Read the model definition and answer for the solid it produces. Units are mm, in the model's axes. A direction names the side the tool comes from. Give positions to 0.01 mm unless a question says otherwise; leave off trailing zeros. Order: outer loops, then holes, each group sorted by start corner. A loop starts at its lowest first (then second) coordinate and runs counter-clockwise, first axis right, second up. Notation, with made-up numbers: (-26.5, 0) - (19.5, 0) arc R20 cw to (19.5, 37) - close; hole circle Ø6 at (5.5, 38). An arc over 180 degrees is marked (long way). Use a Markdown table: item, result. Add a question column.
1. A cutting plane is placed at C-C on x = 1.25. Determine the outline of the cut face in (y, z), and give its area (3 significant figures).
2. A cutting plane is placed at A-A on y = -1.65. Determine the outline of the cut face in (x, z), and give its area (3 significant figures).
3. A cutting plane is placed at D-D on z = 6.75. Determine the outline of the cut face in (x, y).
4. For a pull along X with two mould halves and no side action, classify faces 4 (the flat face through (0, 0, 6)), 5 (the flat face through (19, 2, 3)), 6 (the flat face through (9, 0, 9.7)) as released by +X, released by -X, zero draft, split by the parting line, or undercut.
5. A cutting plane is placed at B-B on z = 4. Determine the outline of the cut face in (x, y), and give its area (3 significant figures).
6. Flat-ended cylindrical pins translate along their axes: P1, Ø1, axis at x = 19, y = 1, coming from the +Z side; P2, Ø1.5, axis at x = 7.5, y = -0.5, coming from the +Z side; P3, Ø2, axis at x = 18.5, z = 4.5, coming from the +Y side. Find the tip coordinate at first contact, or state that the pin passes through.
7. Which of the six approach directions +Z, -Z, +X, -X, +Y, -Y give full straight-line access (tool end or side, diameter ignored) to faces 1 (the flat face through (19, 0, 9)), 2 (the flat face through (19, -2.5, 6)), 3 (the flat face through (19, -2, 3))?
8. Consider L1, parallel to Z at x = 19.25, y = 1.3; L2, parallel to Y at x = 1.5, z = 5.5; L3, parallel to Z at x = 12.75, y = -2.5. Determine where each line is inside the solid, lowest interval first.
```python
from build123d import *

# Parameters (mm, degrees)
PAD_DEPTH         = 20
POCKET_DEPTH      = 2.951
POCKET_DEPTH_BACK = -2.951
PAD001_DEPTH      = 2
PAD002_DEPTH      = 0.7


with BuildPart() as part:
    # Sketch → Pad (new body)
    with BuildSketch(Plane.YZ):
        Polygon((-2.95, 0), (-2.95, 1.4), (-0.7, 1.4), (-0.7, 14.4), (0.7, 14.4), (0.7, 1.4), (2.95, 1.4), (2.95, 0), align=None)
    extrude(amount=PAD_DEPTH)

    # Sketch002 → Pocket (cut, two sides)
    with BuildSketch(Plane.XZ) as pocket_sk:
        Polygon((20, 14.4), (2.290965, 14.4), (20, 2), align=None)
    extrude(amount=-POCKET_DEPTH, mode=Mode.SUBTRACT)
    extrude(pocket_sk.sketch, amount=-POCKET_DEPTH_BACK, mode=Mode.SUBTRACT)

    # Sketch001 (on DatumPlane) → Pad001 (join)
    with BuildSketch(Plane.YZ.offset(20)):
        Polygon((-2.5, 9), (2.5, 9), (2.5, 3), (0.7, 3), (0.7, 1.4), (-0.7, 1.4), (-0.7, 3), (-2.5, 3), align=None)
    extrude(amount=-PAD001_DEPTH)

    # Sketch003 → Pad002 (join, symmetric)
    with BuildSketch(Plane.XZ):
        Polygon((20, 3), (14, 3), (20, 9), align=None)
    extrude(amount=PAD002_DEPTH, both=True)


solid = part.part
```
Output values:
| question | item | result |
|---|---|---|
| 1 | outline | (-2.95, 0) - (2.95, 0) - (2.95, 1.4) - (0.7, 1.4) - (0.7, 14.4) - (-0.7, 14.4) - (-0.7, 1.4) - (-2.95, 1.4) - close |
| 1 | area | 26.5 mm² |
| 2 | outline | (0, 0) - (20, 0) - (20, 1.4) - (0, 1.4) - close; (18, 3) - (20, 3) - (20, 9) - (18, 9) - close |
| 2 | area | 40.0 mm² |
| 3 | outline | (0, -0.7) - (13.22, -0.7) - (13.22, 0.7) - (0, 0.7) - close; (17.75, -0.7) - (18, -0.7) - (18, -2.5) - (20, -2.5) - (20, 2.5) - (18, 2.5) - (18, 0.7) - (17.75, 0.7) - close |
| 4 | face 4 | released by -X |
| 4 | face 5 | zero draft |
| 4 | face 6 | undercut |
| 5 | outline | (0, -0.7) - (18, -0.7) - (18, -2.5) - (20, -2.5) - (20, 2.5) - (18, 2.5) - (18, 0.7) - (0, 0.7) - close |
| 5 | area | 35.2 mm² |
| 6 | P1 | z = 9 |
| 6 | P2 | z = 11.28 |
| 6 | P3 | y = 2.5 |
| 7 | face 1 | +Z, +X, +Y, -Y |
| 7 | face 2 | +Z, +X, -X, -Y |
| 7 | face 3 | +X, -X, -Y |
| 8 | L1 | 0 to 1.4, 3 to 9 |
| 8 | L2 | -0.7 to 0.7 |
| 8 | L3 | 0 to 1.4 |
